Geometry: see drawing. Coordinates: mm, zero at the bounding-box minimum. A direction names the side the tool comes from. Round coordinates to 2 decimals unless told otherwise and drop trailing zeros. Order: outer loops, then holes, each group sorted by start corner. A loop starts at its lowest first (then second) coordinate and runs counter-clockwise, first axis right, second up. Notation, with made-up numbers: (82.5, 25) -> (127.5, 25) arc R20 ccw to (127.5, 36) -> close; hole circle Ø2 at (31, 85.25). An arc over 180 degrees is marked (long way). Put each result on its own line as item: value.
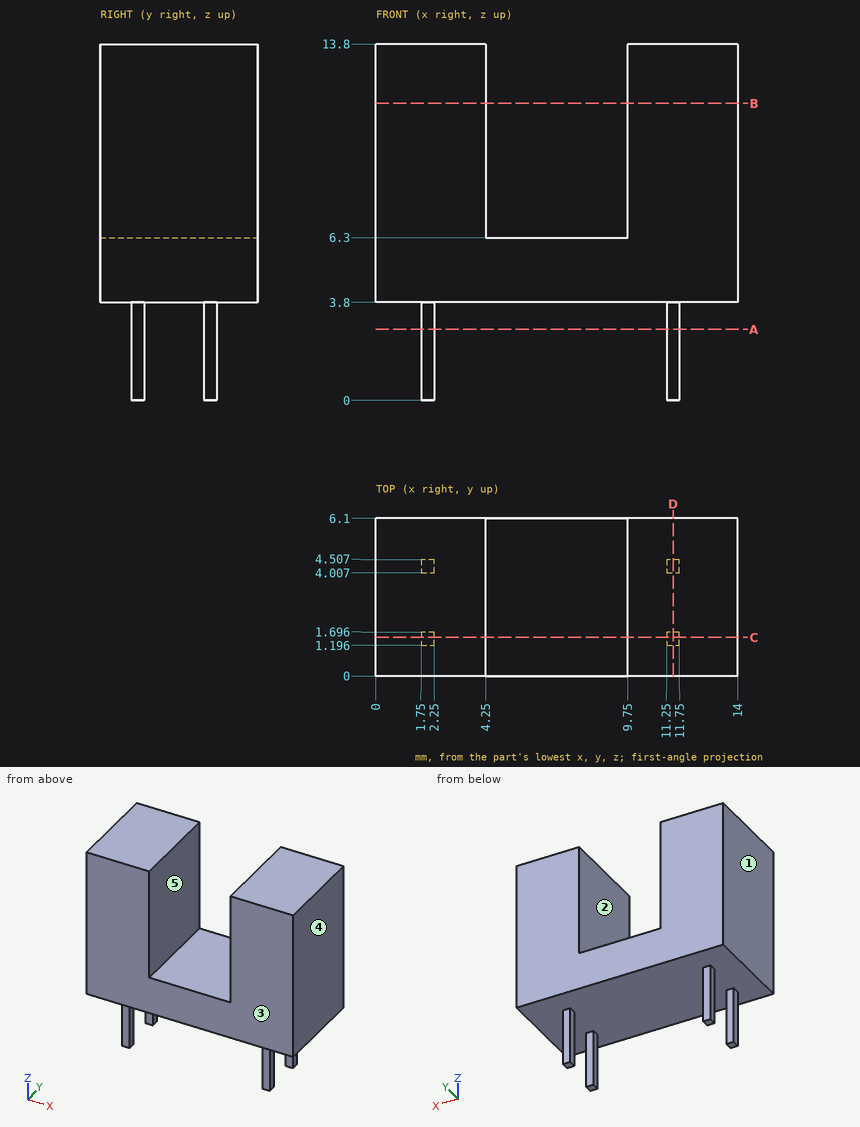
1. Cut plane B-B on z = 11.5. Return loops of the section in (x, y).
Ans:
outline: (0, 0) -> (4.25, 0) -> (4.25, 6.1) -> (0, 6.1) -> close; (9.75, 0) -> (14, 0) -> (14, 6.1) -> (9.75, 6.1) -> close
2. Material intervals for probe 1 along X at (y, z) = (0.5, 13); probe 2 along Z at (x, y) = (2.5, 0.5); probe 3 along Z at (x, y) = (7.75, 0.5), sorted ascending.
Ans:
probe 1: 0 to 4.25, 9.75 to 14
probe 2: 3.8 to 13.8
probe 3: 3.8 to 6.3
3. Cut plane D-D on x = 11.5. Return loops of the section in (y, z).
Ans:
outline: (0, 3.8) -> (1.2, 3.8) -> (1.2, 0) -> (1.7, 0) -> (1.7, 3.8) -> (4.01, 3.8) -> (4.01, 0) -> (4.51, 0) -> (4.51, 3.8) -> (6.1, 3.8) -> (6.1, 13.8) -> (0, 13.8) -> close
4. Contact query for flat-ended pins moving along their axis: P1, Ø2, axis at x = 8, y = 2, coming from the +Z side; P2, Ø0.6, axis at y = 4.5, z = 2, coming from the +X side; P3, Ø2, axis at x = 5.5, z = 9.5, coming from the +Y side; P4, Ø0.6, axis at x = 11.5, z = 2.5, coming from the -Y side. Output: stop coordinate, or through.
Ans:
P1: z = 6.3
P2: x = 11.75
P3: through
P4: y = 1.2
5. Cut plane C-C on y = 1.5. Return loops of the section in (x, z).
Ans:
outline: (0, 3.8) -> (1.75, 3.8) -> (1.75, 0) -> (2.25, 0) -> (2.25, 3.8) -> (11.25, 3.8) -> (11.25, 0) -> (11.75, 0) -> (11.75, 3.8) -> (14, 3.8) -> (14, 13.8) -> (9.75, 13.8) -> (9.75, 6.3) -> (4.25, 6.3) -> (4.25, 13.8) -> (0, 13.8) -> close
6. Cut plane A-A on z = 2.75. Return loops of the section in (x, y), and give its area (3 significant figures).
Ans:
outline: (1.75, 1.2) -> (2.25, 1.2) -> (2.25, 1.7) -> (1.75, 1.7) -> close; (1.75, 4.01) -> (2.25, 4.01) -> (2.25, 4.51) -> (1.75, 4.51) -> close; (11.25, 1.2) -> (11.75, 1.2) -> (11.75, 1.7) -> (11.25, 1.7) -> close; (11.25, 4.01) -> (11.75, 4.01) -> (11.75, 4.51) -> (11.25, 4.51) -> close
area: 1.00 mm²
7. Draft query along X for the marked faces 3, 4 and 5. Return one class per face: +X half, -X half, draft (parallel to the pull), parting line (faces both ways), or undercut.
Ans:
face 3: draft
face 4: +X half
face 5: undercut
8. Set-up query: the marked faces 1 and 2. Return all of +Z, -Z, +X, -X, +Y, -Y with unobstructed straight access to the full face (end or side cutting, diameter ignored); none if empty.
Ans:
face 1: +Z, -Z, -X, +Y, -Y
face 2: +Z, +Y, -Y
